Check sheet for the modelled part. Datum: model origin and axes. Units: mm. A direction names the side the tool comes from. Coordinates: 2 decimals unless noted, no trailing zeros. Loops run counter-clockwise (first coordinate to the right, second up) from the corner with the lowest first, then second, coordinate; pieces in that order, holes last. Notation, with made-up numbers: (-29.5, -14) -> (17.5, -14) arc R29 ccw to (17.5, 23) -> close; hole circle Ø3 at (35, -15). An arc over 180 degrees is marked (long way). Use CSV: the item, a comma, the result in double quotes.
```python
from build123d import *

# Parameters (mm, degrees)
CYLINDER056_R     = 1.75
CYLINDER056_DEPTH = 15
CYLINDER049_R     = 1.75
CYLINDER049_DEPTH = 15
EXTRUDE002_DEPTH  = 4


with BuildPart() as m3holds024:
    # Cylinder056 → Cylinder056 (new body)
    with BuildSketch(Plane(origin=(72, 0.25, 82), x_dir=(1, 0, 0), z_dir=(0, -1, 0))):
        Circle(CYLINDER056_R)
    extrude(amount=CYLINDER056_DEPTH)


with BuildPart() as fusion062:
    # Cylinder049 → Cylinder049 (new body)
    with BuildSketch(Plane(origin=(63.6, 0.25, 61.5), x_dir=(1, 0, 0), z_dir=(0, -1, 0))):
        Circle(CYLINDER049_R)
    extrude(amount=CYLINDER049_DEPTH)

    # Fusion062: union m3Holds024
    add(m3holds024.part)


with BuildPart() as c4holdtopright:
    # Sketch004 → Extrude002 (new body)
    with BuildSketch(Plane.XZ):
        with BuildLine():
            Line((62.586749, 65.351379), (65.538803, 65.351379))
            Line((65.538803, 65.351379), (69.00193, 79))
            Line((69.00193, 79), (69.00193, 84.396622))
            Line((70.021072, 84.435017), (69.00193, 84.396622))
            ThreePointArc((70.021072, 84.435017), (70.953835, 84.821381), (71.340198, 85.754143))
            Line((71.340198, 85.754143), (71.340198, 86.648129))
            ThreePointArc((76.999515, 79), (75.430844, 83.757146), (71.340198, 86.648129))
            Line((76.999515, 79), (76.999515, 71.156998))
            Line((76.999515, 71.156998), (65.547958, 57.96986))
            ThreePointArc((62.586749, 65.351379), (59.954558, 60.010709), (65.547958, 57.96986))
        make_face()
    extrude(amount=EXTRUDE002_DEPTH)


with BuildPart() as c4holdtopright_1:
    # Extrude002 placement: moved
    add(c4holdtopright.part.moved(Location((0, -8, 0))))

    # Cut012: cut Fusion062
    add(fusion062.part, mode=Mode.SUBTRACT)


solid = c4holdtopright_1.part
```
1) Cross-section at C-C on y = -10. Record the boundary of the cut face in (x, z).
Answer below:
outline,"(62.59, 65.35) arc R4 ccw (long way) to (65.55, 57.97) -> (77, 71.16) -> (77, 79) arc R8 ccw to (71.34, 86.65) -> (71.34, 85.75) arc R1.32 cw to (70.02, 84.44) -> (69, 84.4) -> (69, 79) -> (65.54, 65.35) -> close; hole circle Ø3.5 at (63.6, 61.5); hole circle Ø3.5 at (72, 82)"
2) Cross-section at D-D on z = 78. Record the boundary of the cut face in (x, y).
Answer below:
outline,"(68.75, -12) -> (77, -12) -> (77, -8) -> (68.75, -8) -> close"
3) Thickness scan on line 1 along Z through (x, y) = (63.6, -10.8); line 2 along Z through (x, y) = (72, -9.05); line 3 along X through (y, z) = (-10.65, 82.75). Record the ranges inside material, lowest first. Write a range as from..to.
Answer below:
line 1,"z = 57.5..59.75, 63.25..65.35"
line 2,"z = 65.4..80.25, 83.75..86.41"
line 3,"x = 69..70.42, 73.58..76.07"
4) Draft check along X on faces 3 (the cylindrical face through (73.617, -9.972, 81.33)), 4 (the flat face through (71.34, -10, 86)), 5 (the flat face through (64, -10, 65.351)), 6 (the flat face through (71.354, -9.972, 64.656)). Enter one of: released by +X, released by -X, zero draft, split by the parting line, or undercut.
Answer below:
face 3,"undercut"
face 4,"released by -X"
face 5,"zero draft"
face 6,"released by +X"
5) Access from +Z, -Z, +X, -X, +Y, -Y to the whole of each face (thin tool, end or side, straight path). Record for faces 1 (the cylindrical face through (75.473, -9.972, 83.7)), 2 (the flat face through (69.002, -10, 82)).
Answer below:
face 1,"+Z, +X, +Y, -Y"
face 2,"+Z, -X, +Y, -Y"
6) Cross-section at A-A on z = 82. Record the boundary of the cut face in (x, y).
Answer below:
outline,"(69, -12) -> (70.25, -12) -> (70.25, -8) -> (69, -8) -> close; (73.75, -12) -> (76.42, -12) -> (76.42, -8) -> (73.75, -8) -> close"
7) Go/stop test with flat-tipped pins: pin 1 Ø3 at (x, z) = (72, 82) entering from -Y; pin 2 Ø0.9 at (x, y) = (64.5, -10.5) entering from +Z; pin 3 Ø2 at (y, z) = (-10.5, 80.5) entering from -X; pin 4 Ø1 at (y, z) = (-9, 86) entering from -X. Record where each tip stops, or that it passes through.
Answer below:
pin 1,"passes through"
pin 2,"stops at z = 65.35"
pin 3,"stops at x = 69"
pin 4,"stops at x = 71.32"
8) Cross-section at B-B on x = 63.6. Record the boundary of the cut face in (y, z).
Answer below:
outline,"(-12, 57.5) -> (-8, 57.5) -> (-8, 59.75) -> (-12, 59.75) -> close; (-12, 63.25) -> (-8, 63.25) -> (-8, 65.35) -> (-12, 65.35) -> close"
